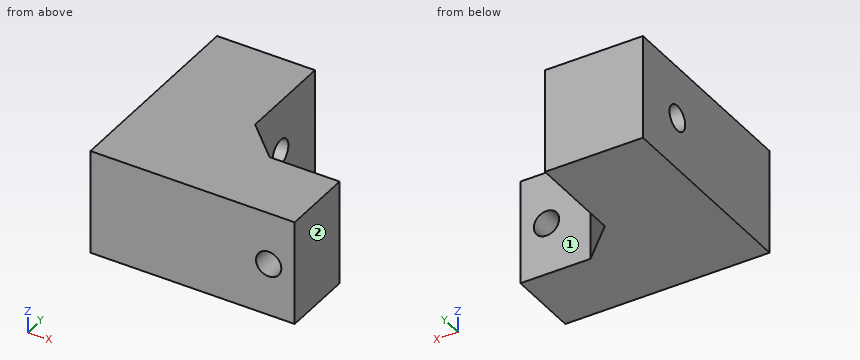
```python
from build123d import *

# Parameters (mm, degrees)
F0_W     = 11.43
F0_H     = 15.24
F0_W_2   = 4.0305707882
F1_DEPTH = 16.51
F3_D     = 4
F5_D     = 4


with BuildPart() as f1:
    # F0 (on Top) → F1 (new body)
    with BuildSketch(Plane.XY):
        Polygon((-32.258, 0), (0, 0), (0, 11.43), (-11.0645864088, 11.43), (-16.7974292118, 17.018), (-20.828, 17.018), (-32.258, 17.018), align=None)
        with Locations((-26.543, 24.638)):
            Rectangle(F0_W, F0_H)
        with Locations((-18.8127146059, 24.638)):
            Rectangle(F0_W_2, F0_H)
    extrude(amount=F1_DEPTH)

    # F3 (through all)
    with Locations(Plane.XZ):
        with Locations((-4.1148, 8.255)):
            Hole(F3_D / 2)

    # F5 (through all)
    with Locations(Plane(origin=(-32.258, 0, 0), x_dir=(0, -1, 0), z_dir=(-1, 0, 0))):
        with Locations((-23.495, 8.255)):
            Hole(F5_D / 2)


solid = f1.part
```
Verification items for the finished model (mm, model axes). Face numbers are marked on the shaded views. A direction names the side the tool comes from. Round coordinates to 2 decimals unless told otherwise and drop trailing zeros. Order: outer loops, then holes, each group sorted by start corner. A loop starts at its lowest first (then second) coordinate and runs counter-clockwise, first axis right, second up.
1) Tool access check on the marked faces 1 and 2. Record the directions out of +Z, -Z, +X, -X, +Y, -Y that give a thin tool (end or side, any length) a straight path to the whole face; none if there is none.
Geometry says:
face 1: +Z, -Z, +X, +Y
face 2: +Z, -Z, +X, +Y, -Y
2) Cross-section at A-A, the plane y = 24. Record the cut outline in (x, z).
Geometry says:
outline: (-32.26, 0) - (-16.8, 0) - (-16.8, 6.32) - (-32.26, 6.32) - close; (-32.26, 10.19) - (-16.8, 10.19) - (-16.8, 16.51) - (-32.26, 16.51) - close
3) Material ranges on line 1 (X direction, y = 28, z = 3.25); line 2 (Z direction, x = -19, y = 25); line 3 (Y direction, x = -7, z = 7.25), recorded low to high.
Geometry says:
line 1: x = -32.26 to -16.8
line 2: z = 0 to 6.94, 9.57 to 16.51
line 3: y = 0 to 11.43
4) Cross-section at C-C, the plane x = -7.5. Record the cut outline in (y, z).
Geometry says:
outline: (0, 0) - (11.43, 0) - (11.43, 16.51) - (0, 16.51) - close
5) Depth check by flat-ended pin: pin 1 (4.5 mm diameter, centred on y = 27, z = 12, fed in from +X); pin 2 (4 mm diameter, centred on x = -7, z = 3.5, fed in from +Y); pin 3 (8 mm diameter, centred on x = -11.5, y = 25, fed in from -Z). Enter the tip coordinate at first touch or a pass-through.
Geometry says:
pin 1: stops at x = -16.8
pin 2: stops at y = 11.43
pin 3: passes through
6) Cross-section at D-D, the plane y = 3.5. Record the cut outline in (x, z) (3 decimals).
Geometry says:
outline: (-32.258, 0) - (0, 0) - (0, 16.51) - (-32.258, 16.51) - close; hole circle Ø4 at (-4.115, 8.255)
7) Cross-section at B-B, the plane z = 11. Record the cut outline in (x, y).
Geometry says:
outline: (-32.26, 0) - (0, 0) - (0, 11.43) - (-11.06, 11.43) - (-16.8, 17.02) - (-16.8, 32.26) - (-32.26, 32.26) - close
